Here's how the part is built. I have some questions about the finished solid (model axes, mm). Face numbers are marked on the shaded views. A direction names the side the tool comes from. Coordinates: 2 decimals unless noted, no trailing zeros. Loops run counter-clockwise (first coordinate to the right, second up) from the corner with the lowest first, then second, coordinate; pieces in that order, holes last. Notation, with made-up numbers: (36, -34.75) -> (43, -34.75) arc R20 cw to (43, -9.75) -> close; hole circle Ø9 at (43.5, 78.25). An arc over 180 degrees is marked (long way). Answer as a JSON object with one key per item and string values. Group by question number.
Q1. I need wall thicknesses on line 1 (Y direction, x = 0, z = 10.25); line 2 (Z direction, x = 29, y = -27.5); line 3 (Y direction, x = 7.5, z = 43). Which ranges of each line are inside material? Lowest first, please.
Q2. On a 3-axis mill with a long thin cutter (end or side, diameter ignored), from which of +Z, -Z, +X, -X, +Y, -Y can I reach the whole of each face in a straight line? I mean the marked faces 1, 2, 3 and 4. Say none if no direction works.
Q3. Thinking about a two-plate mould opening in Y: for the marked faces 5, 6, 7 and 8, which applies, released by +Y, released by -Y, zero draft, split by the parting line, or undercut?
Q4. I want a section at B-B on y = 0. Write out the boundary of the cut face in (x, z).
Q5. I want a section at A-A on x = 0. Write out the boundary of the cut face in (y, z).
Q6. I want a section at C-C on z = 39.5. Write out the boundary of the cut face in (x, y).
Q7. I'm going to push flat-ended pins straight in: pin 1 (12 mm diameter, centred on x = -36.5, z = 9, fed in from +Y); pin 2 (6 mm diameter, centred on x = -15, z = 47, fed in from +Y); pin 3 (7.5 mm diameter, centred on x = 0, y = -48.98, fed in from -Z). Where does each tip first touch, or does it pass through?
Q8. I want a section at D-D on z = 9. Write out the boundary of the cut face in (x, y), then the cut area to 3 significant figures.
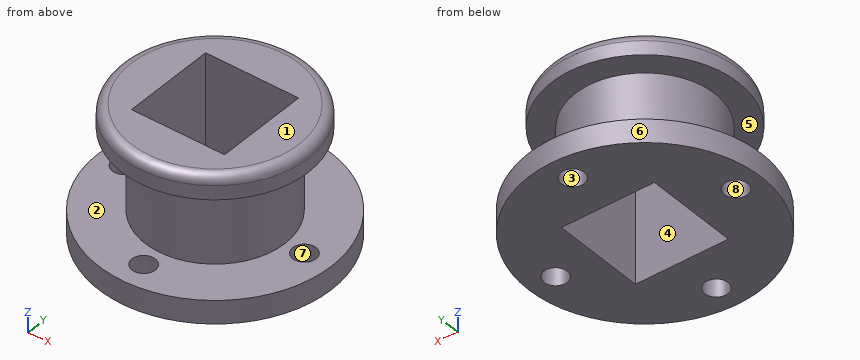
```python
from build123d import *

# Parameters (mm, degrees)
F0_R      = 63.5
F1_DEPTH  = 12.7
F2_R      = 38.1
F3_DEPTH  = 57.15
F4_R      = 6.35
F5_DEPTH  = 12.7
F6_DEPTH  = 25.4
F7_DEPTH  = 25.4
F8_R      = 50.8
F9_DEPTH  = 12.7
F10_W     = 50.8
F10_H     = 50.8
F11_DEPTH = 127
F12_R     = 5.08


with BuildPart() as f1:
    # F0 (on Top) → F1 (new body)
    with BuildSketch(Plane.XY):
        Circle(F0_R)
    extrude(amount=F1_DEPTH)

    # F2 (on Top) → F3 (join)
    with BuildSketch(Plane.XY):
        Circle(F2_R)
    extrude(amount=F3_DEPTH)

    # F4 (on Top) → F5 (cut)
    with BuildSketch(Plane.XY):
        with Locations((-49.74369, 0)):
            Circle(F4_R)
        with Locations((0, 49.552731)):
            Circle(F4_R)
        with Locations((48.788916, 0)):
            Circle(F4_R)
        with Locations((0, -48.979867)):
            Circle(F4_R)
    extrude(amount=-F5_DEPTH, mode=Mode.SUBTRACT)

    # F4 (on Top) → F6 (cut)
    with BuildSketch(Plane.XY):
        with Locations((-49.74369, 0)):
            Circle(F4_R)
        with Locations((0, 49.552731)):
            Circle(F4_R)
        with Locations((48.788916, 0)):
            Circle(F4_R)
        with Locations((0, -48.979867)):
            Circle(F4_R)
    extrude(amount=F6_DEPTH, mode=Mode.SUBTRACT)

    # F4 (on Top) → F7 (cut)
    with BuildSketch(Plane.XY):
        with Locations((-49.74369, 0)):
            Circle(F4_R)
        with Locations((0, 49.552731)):
            Circle(F4_R)
        with Locations((48.788916, 0)):
            Circle(F4_R)
        with Locations((0, -48.979867)):
            Circle(F4_R)
    extrude(amount=-F7_DEPTH, mode=Mode.SUBTRACT)

    # F8 (on face) → F9 (join)
    with BuildSketch(Plane.XY.offset(57.15)):
        Circle(F8_R)
    extrude(amount=F9_DEPTH)

    # F10 (on face) → F11 (cut)
    with BuildSketch(Plane.XY.offset(69.85)):
        Rectangle(F10_W, F10_H)
    extrude(amount=-F11_DEPTH, mode=Mode.SUBTRACT)

    # F12
    f12_edges = [f1.edges().sort_by_distance(p)[0] for p in [
        (-50.8, 0, 69.85),
    ]]
    fillet(f12_edges, radius=F12_R)


solid = f1.part
```
Result set:
{
 "1": {"line 1": "y = -63.5 to -55.33, -42.63 to -25.4, 25.4 to 43.2, 55.9 to 63.5", "line 2": "z = 0 to 12.7, 57.15 to 69.85", "line 3": "y = -37.35 to -25.4, 25.4 to 37.35"},
 "2": {"face 1": "+Z, +X, -X, +Y, -Y", "face 2": "none", "face 3": "-Z", "face 4": "+Z, -Z"},
 "3": {"face 5": "zero draft", "face 6": "split by the parting line", "face 7": "undercut", "face 8": "undercut"},
 "4": {"outline": "(-63.5, 0) -> (-56.09, 0) -> (-56.09, 12.7) -> (-63.5, 12.7) -> close; (-50.8, 57.15) -> (-38.1, 57.15) -> (-38.1, 12.7) -> (-43.39, 12.7) -> (-43.39, 0) -> (-25.4, 0) -> (-25.4, 69.85) -> (-45.72, 69.85) arc R5.08 ccw to (-50.8, 64.77) -> close; (25.4, 0) -> (42.44, 0) -> (42.44, 12.7) -> (38.1, 12.7) -> (38.1, 57.15) -> (50.8, 57.15) -> (50.8, 64.77) arc R5.08 ccw to (45.72, 69.85) -> (25.4, 69.85) -> close; (55.14, 0) -> (63.5, 0) -> (63.5, 12.7) -> (55.14, 12.7) -> close"},
 "5": {"outline": "(-63.5, 0) -> (-55.33, 0) -> (-55.33, 12.7) -> (-63.5, 12.7) -> close; (-50.8, 57.15) -> (-38.1, 57.15) -> (-38.1, 12.7) -> (-42.63, 12.7) -> (-42.63, 0) -> (-25.4, 0) -> (-25.4, 69.85) -> (-45.72, 69.85) arc R5.08 ccw to (-50.8, 64.77) -> close; (25.4, 0) -> (43.2, 0) -> (43.2, 12.7) -> (38.1, 12.7) -> (38.1, 57.15) -> (50.8, 57.15) -> (50.8, 64.77) arc R5.08 ccw to (45.72, 69.85) -> (25.4, 69.85) -> close; (55.9, 0) -> (63.5, 0) -> (63.5, 12.7) -> (55.9, 12.7) -> close"},
 "6": {"outline": "circle Ø76.2 at (0, 0); hole (-25.4, -25.4) -> (25.4, -25.4) -> (25.4, 25.4) -> (-25.4, 25.4) -> close"},
 "7": {"pin 1": "stops at y = 55.7", "pin 2": "stops at y = 36.16", "pin 3": "stops at z = 57.15"},
 "8": {"outline": "circle Ø127 at (0, 0); hole circle Ø12.7 at (-49.74, 0); hole (-25.4, -25.4) -> (25.4, -25.4) -> (25.4, 25.4) -> (-25.4, 25.4) -> close; hole circle Ø12.7 at (0, -48.98); hole circle Ø12.7 at (0, 49.55); hole circle Ø12.7 at (48.79, 0)", "area": "9,580 mm²"}
}
